from build123d import *

# Parameters (mm, degrees)
SKETCH1_R                            = 3.37312
SKETCH1_R_2                          = 14.2875
SKETCH1_R_3                          = 3.3734375
SKETCH1_R_4                          = 2.5527
BASE_FLANGE1_DEPTH                   = 3.175
EDGE_FLANGE1_DEPTH                   = 1016
EDGE_FLANGE2_DEPTH                   = 685.8
EDGE_FLANGE3_STRIP_W                 = 19.05
EDGE_FLANGE3_STRIP_H                 = 3.175
EDGE_FLANGE3_STRIP_CUT_DEPTH         = 158.75
EDGE_FLANGE3_DEPTH                   = 158.75
FILLET1_R                            = 3.175
F_17_64_0_26563_DIAMETER_HOLE1_D     = 6.747002
F_11_32_0_34375_DIAMETER_HOLE1_D     = 8.73125
F_11_32_0_34375_DIAMETER_HOLE2_D     = 8.73125
F_11_32_0_34375_DIAMETER_HOLE2_DEPTH = 3.175
CUT_EXTRUDE2_DEPTH                   = 552.199750341


# Sheet-metal steps are written as plain solids
with BuildPart() as part:
    # Sketch1 → Base-Flange1 (new body)
    with BuildSketch(Plane.XY):
        with BuildLine():
            Line((-481.7491, 38.1), (-481.7491, 82.55))
            Line((-481.7491, 82.55), (-322.9991, 82.55))
            Line((-322.9991, 82.55), (-322.9991, 41.275))
            ThreePointArc((-322.9991, 41.275), (-322.06916403, 39.02993597), (-319.8241, 38.1))
            Line((-319.8241, 38.1), (-319.7987, 38.1))
            ThreePointArc((-319.7987, 38.1), (-317.571596482, 39.022496482), (-316.6491, 41.2496))
            Line((-316.6491, 41.2496), (-316.6491, 41.5036))
            Line((-316.6491, 41.5036), (369.1509, 41.5036))
            Line((369.1509, 41.5036), (369.1509, 41.2496))
            ThreePointArc((369.1509, 41.2496), (370.073396482, 39.022496482), (372.3005, 38.1))
            Line((372.3005, 38.1), (372.3259, 38.1))
            ThreePointArc((372.3259, 38.1), (374.57096403, 39.02993597), (375.5009, 41.275))
            Line((375.5009, 41.275), (375.5009, 82.55))
            Line((375.5009, 82.55), (534.2509, 82.55))
            Line((534.2509, 82.55), (534.2509, 38.1))
            Line((534.2509, 38.1), (534.2509, -38.1))
            Line((534.2509, -38.1), (-481.7491, -38.1))
            Line((-481.7491, -38.1), (-481.7491, 38.1))
        make_face()
        with Locations((-457.073, 0)):
            Circle(SKETCH1_R, mode=Mode.SUBTRACT)
        Circle(SKETCH1_R_2, mode=Mode.SUBTRACT)
        with Locations((-52.5018, 0)):
            Circle(SKETCH1_R_2, mode=Mode.SUBTRACT)
        with Locations((52.5018, 0)):
            Circle(SKETCH1_R_2, mode=Mode.SUBTRACT)
        with Locations((509.5748, 0)):
            Circle(SKETCH1_R, mode=Mode.SUBTRACT)
        with Locations((-93.6625, 30.1625)):
            Circle(SKETCH1_R_3, mode=Mode.SUBTRACT)
        with Locations((93.6625, 30.1625)):
            Circle(SKETCH1_R_3, mode=Mode.SUBTRACT)
        with Locations((93.6625, -30.1625)):
            Circle(SKETCH1_R_3, mode=Mode.SUBTRACT)
        with Locations((-93.6625, -30.1625)):
            Circle(SKETCH1_R_3, mode=Mode.SUBTRACT)
        with Locations((-27.1018, 0)):
            Circle(SKETCH1_R_4, mode=Mode.SUBTRACT)
        with Locations((-52.5018, 25.4)):
            Circle(SKETCH1_R_4, mode=Mode.SUBTRACT)
        with Locations((-52.5018, -25.4)):
            Circle(SKETCH1_R_4, mode=Mode.SUBTRACT)
        with Locations((-77.9018, 0)):
            Circle(SKETCH1_R_4, mode=Mode.SUBTRACT)
    extrude(amount=-BASE_FLANGE1_DEPTH)

    # Edge-Flange1 section (across the edge) → Edge-Flange1 (add)
    with BuildSketch(Plane(origin=(-481.7491, -41.275, 0), x_dir=(0, 1, 0), z_dir=(1, 0, 0))):
        with BuildLine():
            Line((-3.175, 3.175), (-3.175, 47.625))
            Line((-3.175, 47.625), (0, 47.625))
            Line((0, 47.625), (0, 3.175))
            ThreePointArc((0, 3.175), (0.92993597, 0.92993597), (3.175, 0))
            Line((3.175, 0), (3.175, -3.175))
            ThreePointArc((3.175, -3.175), (-1.315128061, -1.315128061), (-3.175, 3.175))
        make_face()
    extrude(amount=EDGE_FLANGE1_DEPTH)

    # Edge-Flange2 section (across the edge) → Edge-Flange2 (add)
    with BuildSketch(Plane(origin=(369.1509, 44.6786, 0), x_dir=(0, -1, 0), z_dir=(-1, 0, 0))):
        with BuildLine():
            Line((-3.175, 3.175), (-3.175, 22.225))
            Line((-3.175, 22.225), (0, 22.225))
            Line((0, 22.225), (0, 3.175))
            ThreePointArc((0, 3.175), (0.92993597, 0.92993597), (3.175, 0))
            Line((3.175, 0), (3.175, -3.175))
            ThreePointArc((3.175, -3.175), (-1.315128061, -1.315128061), (-3.175, 3.175))
        make_face()
    extrude(amount=EDGE_FLANGE2_DEPTH)

    # Edge-Flange3 strip (across the edge) → Edge-Flange3 strip cut (cut)
    with BuildSketch(Plane(origin=(-322.9991, 82.55, 0), x_dir=(0, -1, 0), z_dir=(-1, 0, 0))):
        with Locations((-6.35, -1.5875)):
            Rectangle(EDGE_FLANGE3_STRIP_W, EDGE_FLANGE3_STRIP_H)
    extrude(amount=EDGE_FLANGE3_STRIP_CUT_DEPTH, mode=Mode.SUBTRACT)

    # Edge-Flange3 section (across the edge) → Edge-Flange3 (add)
    with BuildSketch(Plane(origin=(-322.9991, 82.55, 0), x_dir=(0, -1, 0), z_dir=(-1, 0, 0))):
        with BuildLine():
            Line((-3.175, 3.175), (-3.175, 47.625))
            Line((-3.175, 47.625), (0, 47.625))
            Line((0, 47.625), (0, 3.175))
            ThreePointArc((0, 3.175), (0.92993597, 0.92993597), (3.175, 0))
            Line((3.175, 0), (3.175, -3.175))
            ThreePointArc((3.175, -3.175), (-1.315128061, -1.315128061), (-3.175, 3.175))
        make_face()
    extrude(amount=EDGE_FLANGE3_DEPTH)

    # Fillet1
    fillet1_edges = [part.edges().sort_by_distance(p)[0] for p in [
        (-481.7491, -42.8625, 47.625),
        (534.2509, -42.8625, 47.625),
        (369.1509, 46.2661, 22.225),
        (-316.6491, 46.2661, 22.225),
        (-322.9991, 84.1375, 47.625),
        (-481.7491, 84.1375, 47.625),
        (375.5009, 82.55, -1.5875),
        (534.2509, 82.55, -1.5875),
    ]]
    fillet(fillet1_edges, radius=FILLET1_R)

    # 17/64 (0.26563) Diameter Hole1 (through all)
    with Locations(Plane(origin=(0, 0, -3.175), x_dir=(-1, 0, 0), z_dir=(0, 0, -1))):
        with Locations((-324.7009, -22.225), (-324.7009, 22.225), (-172.3009, 22.225), (-172.3009, -22.225), (119.7991, 22.225), (272.1991, 22.225), (272.1991, -22.225), (119.7991, -22.225), (-248.5009, 22.225), (-248.5009, -22.225), (195.9991, 22.225), (195.9991, -22.225)):
            Hole(F_17_64_0_26563_DIAMETER_HOLE1_D / 2)

    # 11/32 (0.34375) Diameter Hole1 (through all)
    with Locations(Plane(origin=(0, 0, -3.175), x_dir=(-1, 0, 0), z_dir=(0, 0, -1))):
        with Locations((-394.5509, 73.025), (-394.5509, 34.925), (-521.5509, 34.925), (-521.5509, 73.025), (342.0491, 34.925), (469.0491, 34.925)):
            Hole(F_11_32_0_34375_DIAMETER_HOLE1_D / 2)

    # 11/32 (0.34375) Diameter Hole2
    with Locations(Plane(origin=(0, 85.725, 0), x_dir=(1, 0, 0), z_dir=(0, 1, 0))):
        with Locations((-465.8741, -25.4), (-338.8741, -25.4)):
            Hole(F_11_32_0_34375_DIAMETER_HOLE2_D / 2, depth=F_11_32_0_34375_DIAMETER_HOLE2_DEPTH)

    # Sketch34 → Cut-Extrude2 (cut, through all)
    with BuildSketch(Plane(origin=(0, -41.275, 0), x_dir=(1, 0, 0), z_dir=(0, 1, 0))):
        with BuildLine():
            Line((-399.1991, -22.0265625), (-386.4991, -22.0265625))
            ThreePointArc((-386.4991, -22.0265625), (-383.1256625, -25.4), (-386.4991, -28.7734375))
            Line((-386.4991, -28.7734375), (-399.1991, -28.7734375))
            ThreePointArc((-399.1991, -28.7734375), (-402.5725375, -25.4), (-399.1991, -22.0265625))
        make_face()
        with BuildLine():
            Line((-107.0991, -28.7734375), (-119.7991, -28.7734375))
            ThreePointArc((-119.7991, -28.7734375), (-123.1725375, -25.4), (-119.7991, -22.0265625))
            Line((-119.7991, -22.0265625), (-107.0991, -22.0265625))
            ThreePointArc((-107.0991, -22.0265625), (-103.7256625, -25.4), (-107.0991, -28.7734375))
        make_face()
        with BuildLine():
            Line((159.6009, -22.0265625), (172.3009, -22.0265625))
            ThreePointArc((172.3009, -22.0265625), (175.6743375, -25.4), (172.3009, -28.7734375))
            Line((172.3009, -28.7734375), (159.6009, -28.7734375))
            ThreePointArc((159.6009, -28.7734375), (156.2274625, -25.4), (159.6009, -22.0265625))
        make_face()
        with BuildLine():
            Line((439.0009, -22.0265625), (451.7009, -22.0265625))
            ThreePointArc((451.7009, -22.0265625), (455.0743375, -25.4), (451.7009, -28.7734375))
            Line((451.7009, -28.7734375), (439.0009, -28.7734375))
            ThreePointArc((439.0009, -28.7734375), (435.6274625, -25.4), (439.0009, -22.0265625))
        make_face()
    extrude(amount=-CUT_EXTRUDE2_DEPTH, mode=Mode.SUBTRACT)


solid = part.part
For this review, take the finished solid that the model builds, in its own axes (mm). A direction names the side the tool comes from. Give positions to 0.01 mm unless a question says otherwise; leave off trailing zeros. Loops run counter-clockwise (first coordinate to the right, second up) from the corner with the lowest first, then second, coordinate; pieces in that order, holes last. Notation, with made-up numbers: (78, 29.25) - (124, 29.25) arc R34 cw to (124, 66.25) - close; hole circle Ø2 at (47, -9). An arc over 180 degrees is marked (long way). Write each question's results on one line, items separated by ' | '.
(1) Take a section at B-B (x = 204.5). Give the boundary of the cut face in (y, z) (3 decimals).
Conclusion:
outline: (-44.45, 3.175) arc R6.35 ccw to (-38.1, -3.175) - (41.504, -3.175) arc R6.35 ccw to (47.854, 3.175) - (47.854, 22.225) - (44.679, 22.225) - (44.679, 3.175) arc R3.175 cw to (41.504, 0) - (-38.1, 0) arc R3.175 cw to (-41.275, 3.175) - (-41.275, 47.625) - (-44.45, 47.625) - close
(2) For line 1 along Y through (x, z) = (-142, 10) (3 decimals); line 2 along Y through (x, z) = (-394.5, 30.5) (3 decimals); line 3 along Z through (x, y) = (-441, -33.5) (3 decimals), list the stretches that pass through material, from the lowest coordinate up.
Conclusion:
line 1: -44.45 to -41.275, 44.679 to 47.854 | line 2: -44.45 to -41.275, 82.55 to 85.725 | line 3: -3.175 to 0
(3) For pin 1 Ø3.5 at (x, y) = (-112.5, -42) entering from -Z; pin 2 Ø1 at (x, y) = (-79.5, 1) entering from -Z; pin 3 Ø4 at (x, z) = (190, 28.5) entering from +Y (3 decimals); pin 4 Ø8 at (x, y) = (261.5, -26) entering from +Z, all flat-tipped, find the tip position at first contact; note any pin that passes through.
Conclusion:
pin 1: z = -2.8 | pin 2: through | pin 3: y = -41.275 | pin 4: z = 0
(4) For faces 1 (the flat face through (-322.999, 83, 10)), 2 (the flat face through (-481.749, 20.3, -0.4)), 3 (the flat face through (-401, 82.55, 26)), list the 3-axis set-ups (+Z, -Z, +X, -X, +Y, -Y) from which the entire face can be reached by the end or side of a thin tool; tool diameter is ignored.
Conclusion:
face 1: +Z, -Z, +Y | face 2: +Z, -Z, -X, +Y, -Y | face 3: +Z, +X, -X
(5) Draft analysis for pull direction X (two halves, no side actions). For faces 4 (the cylindrical face through (-66.775, 0.628, -1.565)), 5 (the flat face through (534.251, -0.6, -0.4)), 6 (the flat face through (-401, 85.725, 25)), state which applies: +X half, -X half, draft (parallel to the pull), parting line (faces both ways), or undercut.
Conclusion:
face 4: undercut | face 5: +X half | face 6: draft
